Geometry: final body of the model. Coordinates: model frame, mm. A direction names the side the tool comes from. Coordinates: 2 decimals unless noted, no trailing zeros. Loops run counter-clockwise (first coordinate to the right, second up) from the corner with the lowest first, then second, coordinate; pieces in that order, holes last. Notation, with made-up numbers: (80.25, -25) -> (120.25, -25) arc R27 cw to (120.25, -9) -> close; hole circle Ø11 at (49, 72.5). An arc over 180 degrees is marked (long way). One line per item, written item: value. Start each with the question number.
Item 1: Section query B-B on y = 2.25. Return loops of the section in (x, z).
Item 2: Mould query, pull axis X, two halves, no side actions, for faces 6 (the flat face through (-2, 14.8, 2)), 7 (the cylindrical face through (0, 13, 2)), 8 (the cylindrical face through (4.64, 1.92, -1.46)). Classes: +X half, -X half, draft (parallel to the pull), parting line (faces both ways), or undercut.
Item 3: Section query A-A on y = 5.75. Return loops of the section in (x, z), then the cut area to 3 significant figures.
Item 4: Contact query for flat-ended pins moving along their axis: pin 1 Ø2 at (y, z) = (11.5, -1.5) entering from -X; pin 2 Ø4 at (y, z) = (14.5, 2.5) entering from +X; pin 3 Ø1 at (y, z) = (3, 0) entering from -X. Output: stop coordinate, or through.
Item 5: Ray query, probe 1 along Y at (x, z) = (3.5, 0); probe 2 along Y at (x, z) = (3.5, -2.5); probe 3 along Y at (x, z) = (-1, 4.5). Return the intervals inside material, ascending. Write a range as from..to.
Item 6: Set-up query: faces 1 (the flat face through (-2.468, 9.683, -4.349)), 2 (the flat face through (5, 10, 0)), 3 (the flat face through (2.468, 9.683, 4.349)), 4 (the cylindrical face through (-0.534, 5.006, -4.065)), 5 (the cylindrical face through (4.88, 17.14, -1.08)). Return all of +Z, -Z, +X, -X, +Y, -Y with unobstructed straight access to the full face (end or side cutting, diameter ignored); none if empty.
Item 7: Section query C-C on y = 11.75. Return loops of the section in (x, z).
from build123d import *

# Parameters (mm, degrees)
ESTRUSIONE_ESTRUSIONE1_START                         = 8
ESTRUSIONE_ESTRUSIONE1_2_OUTLINE_R                   = 4.864
ESTRUSIONE_ESTRUSIONE1_2_DEPTH                       = 3.491917096
SCHIZZO2_R                                           = 4.85
ESTRUSIONE_ESTRUSIONE2_DEPTH                         = 3.3
SCHIZZO3_R                                           = 2.55
ESTRUSIONE_ESTRUSIONE3_DEPTH                         = 1.5
SCHIZZO4_R                                           = 5
ESTRUSIONE_ESTRUSIONE4_DEPTH                         = 1.7
FORO_LAMATO_PER_VITE_M2_5_A_TESTA_ESAGON_D           = 3.1
FORO_LAMATO_PER_VITE_M2_5_A_TESTA_ESAGON_CBORE_D     = 4
FORO_LAMATO_PER_VITE_M2_5_A_TESTA_ESAGON_CBORE_DEPTH = 10
SMUSSO1_SIZE                                         = 0.581


with BuildPart() as part:
    # Estrusione-Estrusione1: read off the stored shape, not the designer's step
    # Estrusione-Estrusione1 outline → Estrusione-Estrusione1 (revolve)
    with BuildSketch(Plane.XY):
        with BuildLine():
            Line((0, 0), (4.864, 0))
            Line((4.864, 0), (4.864, 3.219))
            Line((4.864, 3.219), (4.1, 3.983))
            Line((4.1, 3.983), (4.1, 6))
            ThreePointArc((4.1, 6), (4.99, 5.11), (5.88, 6))
            Line((5.88, 6), (7, 6))
            Line((7, 6), (7, 8))
            Line((7, 8), (4.864, 8))
            Line((4.864, 8), (4.864, 11.491917096))
            Line((4.864, 11.491917096), (4.85, 11.5))
            Line((4.85, 11.5), (0, 11.5))
            Line((0, 11.5), (0, 0))
        make_face()
    revolve(axis=Axis((0, 0, 0), (0, 1, 0)))

    # Estrusione-Estrusione1 2 outline → Estrusione-Estrusione1 2 (add)
    with BuildSketch(Plane(origin=(0, 0, 0), x_dir=(1, 0, 0), z_dir=(0, 1, 0)).offset(ESTRUSIONE_ESTRUSIONE1_START)):
        with BuildLine():
            ThreePointArc((4.77856863, -3.014594807), (4.893043531, -2.825), (5, -2.631064423))
            Line((5, -2.631064423), (5, 2.631064423))
            ThreePointArc((5, 2.631064423), (4.893043531, 2.825), (4.77856863, 3.014594807))
            Line((4.77856863, 3.014594807), (0.22143137, 5.645659231))
            ThreePointArc((0.22143137, 5.645659231), (0, 5.65), (-0.22143137, 5.645659231))
            Line((-0.22143137, 5.645659231), (-4.77856863, 3.014594807))
            ThreePointArc((-4.77856863, 3.014594807), (-4.893043531, 2.825), (-5, 2.631064423))
            Line((-5, 2.631064423), (-5, -2.631064423))
            ThreePointArc((-5, -2.631064423), (-4.893043531, -2.825), (-4.77856863, -3.014594807))
            Line((-4.77856863, -3.014594807), (-0.22143137, -5.645659231))
            ThreePointArc((-0.22143137, -5.645659231), (0, -5.65), (0.22143137, -5.645659231))
            Line((0.22143137, -5.645659231), (4.77856863, -3.014594807))
        make_face()
        Circle(ESTRUSIONE_ESTRUSIONE1_2_OUTLINE_R, mode=Mode.SUBTRACT)
    extrude(amount=ESTRUSIONE_ESTRUSIONE1_2_DEPTH)

    # Estrusione-Estrusione1 3 outline → Estrusione-Estrusione1 3 (revolve, cut)
    with BuildSketch(Plane.XY):
        Polygon((5.65, 11.491917096), (4.864, 11.491917096), (5.65, 11.038119785), align=None)
    revolve(axis=Axis((0, 0, 0), (0, 1, 0)), mode=Mode.SUBTRACT)

    # Schizzo2 → Estrusione-Estrusione2 (add)
    with BuildSketch(Plane(origin=(0, 11.5, 0), x_dir=(-1, 0, 0), z_dir=(0, 1, 0))):
        with Locations(Location((0, 0, 0), (0, 0, 90))):
            Circle(SCHIZZO2_R)
    extrude(amount=ESTRUSIONE_ESTRUSIONE2_DEPTH)

    # Schizzo3 → Estrusione-Estrusione3 (add)
    with BuildSketch(Plane(origin=(0, 14.8, 0), x_dir=(-1, 0, 0), z_dir=(0, 1, 0))):
        with Locations(Location((0, 0, 0), (0, 0, 270))):
            Circle(SCHIZZO3_R)
    extrude(amount=ESTRUSIONE_ESTRUSIONE3_DEPTH)

    # Schizzo4 → Estrusione-Estrusione4 (add)
    with BuildSketch(Plane.XZ.offset(-16.3)):
        with Locations(Location((0, 0, 0), (0, 0, 90))):
            Circle(SCHIZZO4_R)
    extrude(amount=-ESTRUSIONE_ESTRUSIONE4_DEPTH)

    # Foro lamato per Vite M2.5 a testa esagonale-1 (through all)
    with Locations(Plane(origin=(0, 18, 0), x_dir=(1, 0, 0), z_dir=(0, 1, 0))):
        with Locations((0, 0)):
            CounterBoreHole(FORO_LAMATO_PER_VITE_M2_5_A_TESTA_ESAGON_D / 2, FORO_LAMATO_PER_VITE_M2_5_A_TESTA_ESAGON_CBORE_D / 2, FORO_LAMATO_PER_VITE_M2_5_A_TESTA_ESAGON_CBORE_DEPTH)

    # Smusso1
    smusso1_edges = [part.edges().sort_by_distance(p)[0] for p in [
        (-4.864, 0, 0),
    ]]
    chamfer(smusso1_edges, length=SMUSSO1_SIZE)


solid = part.part
Reply:
1. outline: circle Ø9.73 at (0, 0); hole circle Ø3.1 at (0, 0)
2. face 6: draft
2. face 7: undercut
2. face 8: parting line
3. outline: circle Ø11.69 at (0, 0); circle Ø8.2 at (0, 0); hole circle Ø8.27 at (0, 0); hole circle Ø3.1 at (0, 0)
3. area: 98.8 mm²
4. pin 1: stops at x = -5
4. pin 2: stops at x = 4.82
4. pin 3: stops at x = -4.86
5. probe 1: y = 0..14.8, 16.3..18
5. probe 2: y = 0.02..3.78, 5.44..14.8, 16.3..18
5. probe 3: y = 0.33..3.47, 5.2..14.8, 16.3..18
6. face 1: -Z, -X, +Y
6. face 2: +Z, -Z, +X, +Y
6. face 3: +Z, +X, +Y
6. face 4: none
6. face 5: +Y
7. outline: circle Ø9.7 at (0, 0); hole circle Ø4 at (0, 0)
